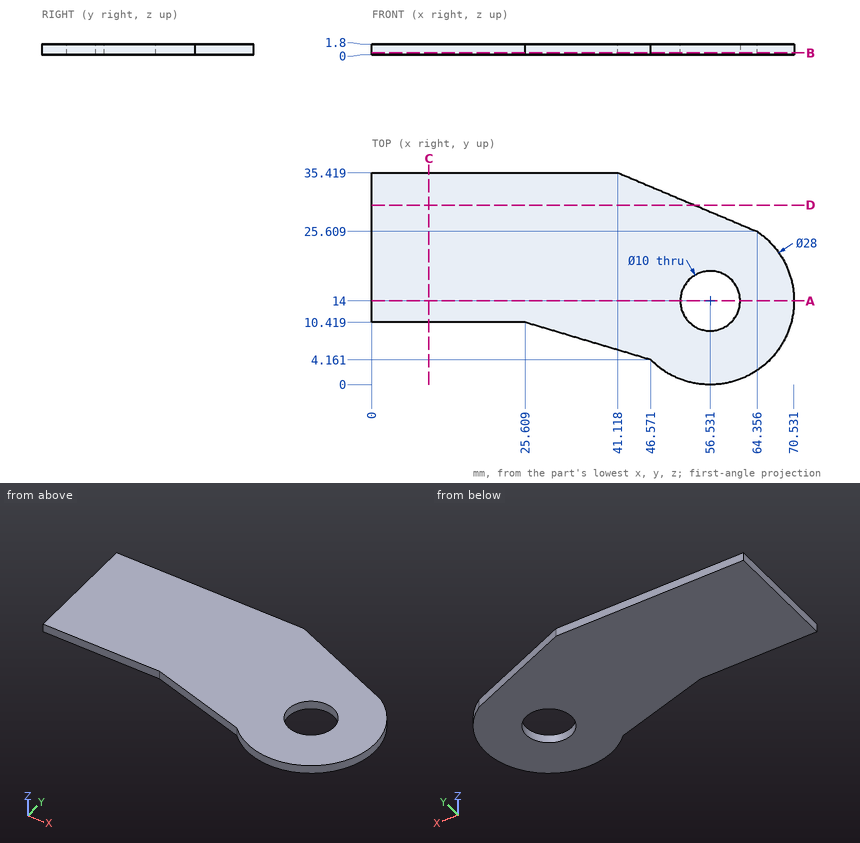
The figure shows three views and two pictorial views of one solid part (mm, origin at its lowest corner). Answer the questions. Give positions to 0.01 mm unless a question says otherwise; leave off trailing zeros. Order: outer loops, then holes, each group sorted by start corner. A loop starts at its lowest first (then second) coordinate and runs counter-clockwise, first axis right, second up. Notation, with made-up numbers: (-18.75, 39) -> (35.25, 39) arc R16 cw to (35.25, 56) -> close; hole circle Ø2 at (34.5, 80). An arc over 180 degrees is marked (long way). Answer as CSV lines item,"result". Start each with the question number.
(1) Consider line 1 along X through (y, z) = (14, 0.9); line 2 along Y through (x, z) = (56, 0.55) (1 decimal); line 3 along Y through (x, z) = (22, 1.3). Determine where each line is inside the solid, lowest interval first.
(2) Section D-D, the plane y = 30 is taken. Write down the section's boundary in (x, z) (1 decimal).
(3) Section B-B, the plane z = 0.3 is taken. Write down the section's boundary in (x, y) (1 decimal).
(4) Section C-C, the plane x = 9.5 is taken. Write down the section's boundary in (y, z).
(5) This flat-tipped pin is pushed along its axis until it touches: pin 1 Ø1 at (x, z) = (11.5, 1.5) entering from -Y. Where does it stop, or does it pass through?
(6) Section A-A, the plane y = 14 is taken. Write down the section's boundary in (x, z), plus the area to 3 significant figures.
Entries:
1,line 1,"0 to 51.53, 61.53 to 70.53"
1,line 2,"0 to 9, 19 to 29.1"
1,line 3,"10.42 to 35.42"
2,outline,"(0, 0) -> (54, 0) -> (54, 1.8) -> (0, 1.8) -> close"
3,outline,"(0, 10.4) -> (25.6, 10.4) -> (46.6, 4.2) arc R14 ccw (long way) to (64.4, 25.6) -> (41.1, 35.4) -> (0, 35.4) -> close; hole circle Ø10 at (56.5, 14)"
4,outline,"(10.42, 0) -> (35.42, 0) -> (35.42, 1.8) -> (10.42, 1.8) -> close"
5,pin 1,"y = 10.42"
6,outline,"(0, 0) -> (51.53, 0) -> (51.53, 1.8) -> (0, 1.8) -> close; (61.53, 0) -> (70.53, 0) -> (70.53, 1.8) -> (61.53, 1.8) -> close"
6,area,"109 mm²"
